Geometry check sheet. Reference: the model listing, model coordinates, mm. A direction names the side the tool comes from. Give positions to 0.01 mm unless a question says otherwise; leave off trailing zeros. Loops run counter-clockwise (first coordinate to the right, second up) from the corner with the lowest first, then second, coordinate; pieces in that order, holes last.
1. Cross-section at B-B, the plane x = -23. Record the cut outline in (y, z), plus the area to 3 significant figures.
2. Material ranges on L1, parallel to Y at x = 0, z = 15.5; L2, parallel to X at y = 0, z = 14; L3, parallel to Z at x = 6.5, y = -2.5, recorded low to high.
3. Cross-section at A-A, the plane y = 0. Record the cut outline in (x, z).
4. Cross-section at D-D, the plane z = 17.5. Record the cut outline in (x, y), plus the area to 3 significant figures.
5. Cross-section at C-C, the plane z = 28. Record the cut outline in (x, y), plus the area to 3 significant figures.
6. Release check for a two-part mould opening along X. For faces 1 (the cylindrical face through (-11.056, 10.138, 20.14)), 2 (the flat face through (0, 0, 0)), 3 (the flat face through (30, -0.3, 14.8)) record: +X half, -X half, draft (parallel to the pull), parting line (faces both ways), or undercut.
7. Tool access check on faces 4 (the flat face through (0, 0, 10)), 5 (the flat face through (-23, 0, 15)), 6 (the flat face through (0, 25, 15)). Record the directions out of +Z, -Z, +X, -X, +Y, -Y that give a thin tool (end or side, any length) a straight path to the whole face; none if there is none.
from build123d import *

# Parameters (mm, degrees)
SKETCH_W        = 60
SKETCH_H        = 50
PAD_DEPTH       = 30
SKETCH001_R     = 15
POCKET_DEPTH    = 20
POCKET001_DEPTH = 60.001
FILLET_R        = 5


with BuildPart() as part:
    # Sketch → Pad (new body)
    with BuildSketch(Plane.XY):
        Rectangle(SKETCH_W, SKETCH_H)
    extrude(amount=PAD_DEPTH)

    # Sketch001 (on Face6 of Pad) → Pocket (cut)
    with BuildSketch(Plane.XY.offset(30)):
        Circle(SKETCH001_R)
    extrude(amount=-POCKET_DEPTH, mode=Mode.SUBTRACT)

    # Sketch002 (on Face3 of Pocket) → Pocket001 (cut, through all)
    with BuildSketch(Plane.YZ.offset(30)):
        with BuildLine():
            ThreePointArc((10, 15), (0, 25), (-10, 15))
            Line((-10, 15), (10, 15))
        make_face()
    extrude(amount=-POCKET001_DEPTH, mode=Mode.SUBTRACT)

    # Fillet
    fillet_edges = [part.edges().sort_by_distance(p)[0] for p in [
        (0, -25, 30),
    ]]
    fillet(fillet_edges, radius=FILLET_R)


solid = part.part
Result:
1. outline: (-25, 0) - (25, 0) - (25, 30) - (-20, 30) arc R5 ccw to (-25, 25) - close; hole (-10, 15) - (10, 15) arc R10 ccw to start
1. area: 1,340 mm2
2. L1: y = -25 to -15, 15 to 25
2. L2: x = -30 to -15, 15 to 30
2. L3: z = 0 to 10
3. outline: (-30, 0) - (30, 0) - (30, 15) - (15, 15) - (15, 10) - (-15, 10) - (-15, 15) - (-30, 15) - close; (-30, 25) - (-15, 25) - (-15, 30) - (-30, 30) - close; (15, 25) - (30, 25) - (30, 30) - (15, 30) - close
4. outline: (-30, -25) - (30, -25) - (30, -9.68) - (11.46, -9.68) arc R15 cw to (-11.46, -9.68) - (-30, -9.68) - close; (-30, 9.68) - (-11.46, 9.68) arc R15 cw to (11.46, 9.68) - (30, 9.68) - (30, 25) - (-30, 25) - close
4. area: 1,670 mm2
5. outline: (-30, -24) - (30, -24) - (30, 25) - (-30, 25) - close; hole circle Ø30 at (0, 0)
5. area: 2,230 mm2
6. face 1: undercut
6. face 2: draft
6. face 3: +X half
7. face 4: +Z
7. face 5: +X, -X
7. face 6: +Z, -Z, +X, -X, +Y
